from build123d import *

# Parameters (mm, degrees)
SKETCH1_W           = 76.2
SKETCH1_H           = 88.9
BOSS_EXTRUDE1_DEPTH = 73.025
BOSS_EXTRUDE2_DEPTH = 4.7625
FILLET1_R           = 2.54
CUT_EXTRUDE1_DEPTH  = 5.7625
FILLET2_R           = 2.54
SKETCH4_R           = 2.1
CUT_EXTRUDE2_DEPTH  = 25.4


with BuildPart() as part:
    # Sketch1 → Boss-Extrude1 (new body)
    with BuildSketch(Plane(origin=(0, 0, 0), x_dir=(1, 0, 0), z_dir=(0, 1, 0))):
        with Locations((38.1, 44.45)):
            Rectangle(SKETCH1_W, SKETCH1_H)
    extrude(amount=BOSS_EXTRUDE1_DEPTH)

    # Sketch2 → Boss-Extrude2 (add)
    with BuildSketch(Plane.XZ):
        Polygon((38.1, 0), (38.1, 19.05), (95.25, 19.05), (95.25, -107.95), (38.1, -107.95), (38.1, -88.9), align=None)
    extrude(amount=-BOSS_EXTRUDE2_DEPTH)

    # Fillet1
    fillet1_edges = [part.edges().sort_by_distance(p)[0] for p in [
        (38.1, 2.38125, -107.95),
        (38.1, 2.38125, 19.05),
        (95.25, 2.38125, 19.05),
        (95.25, 2.38125, -107.95),
        (0, 36.5125, -88.9),
        (76.2, 38.89375, -88.9),
        (76.2, 38.89375, 0),
        (0, 36.5125, 0),
    ]]
    fillet(fillet1_edges, radius=FILLET1_R)

    # Sketch3 → Cut-Extrude1 (cut, through all)
    with BuildSketch(Plane(origin=(0, 4.7625, 0), x_dir=(1, 0, 0), z_dir=(0, 1, 0))):
        with BuildLine():
            Line((45.796852287, 99.655), (85.725, 99.655))
            ThreePointArc((85.725, 99.655), (88.225, 97.155), (85.725, 94.655))
            Line((85.725, 94.655), (45.796852287, 94.655))
            ThreePointArc((45.796852287, 94.655), (43.296852287, 97.155), (45.796852287, 99.655))
        make_face()
        with BuildLine():
            Line((45.796852287, -10.755), (85.725, -10.755))
            ThreePointArc((85.725, -10.755), (88.225, -8.255), (85.725, -5.755))
            Line((85.725, -5.755), (45.796852287, -5.755))
            ThreePointArc((45.796852287, -5.755), (43.296852287, -8.255), (45.796852287, -10.755))
        make_face()
        with BuildLine():
            Line((88.225, 86.36), (88.225, 2.54))
            ThreePointArc((88.225, 2.54), (85.725, 0.04), (83.225, 2.54))
            Line((83.225, 2.54), (83.225, 86.36))
            ThreePointArc((83.225, 86.36), (85.725, 88.86), (88.225, 86.36))
        make_face()
    extrude(amount=-CUT_EXTRUDE1_DEPTH, mode=Mode.SUBTRACT)

    # Fillet2
    fillet2_edges = [part.edges().sort_by_distance(p)[0] for p in [
        (55.88, 4.7625, -88.9),
        (38.1, 2.38125, 0),
        (38.1, 2.38125, -88.9),
        (76.2, 4.7625, -44.45),
        (55.88, 4.7625, 0),
        (75.456051224, 4.7625, -88.156051224),
        (75.456051224, 4.7625, -0.743948776),
    ]]
    fillet(fillet2_edges, radius=FILLET2_R)

    # Sketch4 → Cut-Extrude2 (cut)
    with BuildSketch(Plane(origin=(0, 73.025, 0), x_dir=(1, 0, 0), z_dir=(0, 1, 0))):
        with Locations((12.303125, 78.58125)):
            Circle(SKETCH4_R)
        with Locations((12.303125, 10.31875)):
            Circle(SKETCH4_R)
        with Locations((63.896875, 10.31875)):
            Circle(SKETCH4_R)
        with Locations((63.896875, 78.58125)):
            Circle(SKETCH4_R)
    extrude(amount=-CUT_EXTRUDE2_DEPTH, mode=Mode.SUBTRACT)


solid = part.part
Verification items for the finished model (mm, model axes). A direction names the side the tool comes from. Coordinates: 2 decimals unless noted, no trailing zeros. Write each loop counter-clockwise with the first axis right and the second up, starting at its lowest first coordinate (ties: lowest second). Pieces come first, ordered by that corner, then holes. Notation, with made-up numbers: M 66.25,38 L 94.25,38 A24 cw 94.25,73 Z; hole C 67.25,24.25 d4. An arc over 180 degrees is marked long. Use CSV: the item, a comma, the result in double quotes.
Q1. Section check B-B, the plane x = 51.5. State how many separate pieces and enclosed holes the cut face has, and give its area (3 significant figures).
Computed values:
separate pieces,"3"
enclosed holes,"0"
area,"6,630 mm²"
Q2. Thickness scan on line 1 along Z through (x, y) = (54.5, 53.5); line 2 along X through (y, z) = (16.5, -75); line 3 along Y through (x, z) = (76, 0). Record the ranges inside material, lowest first. Write a range as [from, to].
Computed values:
line 1,"[-88.9, 0]"
line 2,"[0, 76.2]"
line 3,"[0, 5.35]"
Q3. Section check C-C, the plane y = 37. Enter the section's corners in (x, z).
Computed values:
outline,"M 0,-86.36 A2.54 ccw 2.54,-88.9 L 73.66,-88.9 A2.54 ccw 76.2,-86.36 L 76.2,-2.54 A2.54 ccw 73.66,0 L 2.54,0 A2.54 ccw 0,-2.54 Z"
Q4. Set-up check for faces 1 (the flat face through (64, 47.625, -10)), 2 (the flat face through (38.1, 2, -98)), 3 (the flat face through (76.2, 40, -44)), 4 (the cylindrical face through (85.78, 2.41, -0.04)): record each of +Z, -Z, +X, -X, +Y, -Y from which the full face is reachable in a straight line by a thin tool's end or side.
Computed values:
face 1,"+Y"
face 2,"-Z, -X, +Y, -Y"
face 3,"+Z, -Z, +X, +Y"
face 4,"+Y, -Y"
Q5. Mould release check, pull along Z, two halves, no side actions. Record for faces 5 (the flat face through (80, 4.762, -44)), 6 (the cylindrical face through (88.224, 2.415, -97.21)), 7 (the flat face through (66, 2, 19.05)), 8 (the cylindrical face through (65.03, 60.5, -80.35)): pulls with the +Z half, pulls with the -Z half, needs draft (parallel to the pull), parting line crosses it, or undercut.
Computed values:
face 5,"needs draft"
face 6,"undercut"
face 7,"pulls with the +Z half"
face 8,"undercut"
Q6. Section check D-D, the plane y = 56. Enter the section's corners in (x, z).
Computed values:
outline,"M 0,-86.36 A2.54 ccw 2.54,-88.9 L 73.66,-88.9 A2.54 ccw 76.2,-86.36 L 76.2,-2.54 A2.54 ccw 73.66,0 L 2.54,0 A2.54 ccw 0,-2.54 Z; hole C 12.3,-78.58 d4.2; hole C 12.3,-10.32 d4.2; hole C 63.9,-78.58 d4.2; hole C 63.9,-10.32 d4.2"
Q7. Go/stop test with flat-tipped pins: P1, Ø5, axis at y = 54, z = -80, coming from the +X side; P2, Ø2.5, axis at x = 63.9, z = -78.58, coming from the +Y side (3 decimals); P3, Ø10, axis at x = 62.5, y = 39.5, coming from the -Z side. Record where each tip stops, or that it passes through.
Computed values:
P1,"x = 76.2"
P2,"y = 47.625"
P3,"z = -88.9"
